Geometry: final body of the model. Coordinates: model frame, mm. A direction names the side the tool comes from. Give positions to 0.01 mm unless a question says otherwise; leave off trailing zeros. Order: outer loops, then holes, each group sorted by start corner. A loop starts at its lowest first (then second) coordinate and runs counter-clockwise, first axis right, second up. Notation, with made-up numbers: (35.5, 73) - (70.5, 73) arc R8 ccw to (70.5, 80) - close; hole circle Ø5 at (60.5, -27.75). An arc over 180 degrees is marked (long way). One line per question, with ' | ' between items. Start each with the question number.
Autodesk Fusion 360 part; units mm, degrees
sketch "Sketch1" plane through (0, 0, 0) normal (0, 1, 0) x (1, 0, 0)
  line L0 (30, 40) -> (-120, 40)
  line L1 (-120, 40) -> (-120, 20)
  line L2 (-120, 20) -> (-30, 20)
  line L3 (-30, 20) -> (-30, 0)
  arc A0 (-30, 0) -> (30, 0) centre (0, 0) ccw
  line L4 (30, 0) -> (30, 40)
  dimension "d3" = 30
  dimension "d4" = 150
  dimension "d5" = 20
  dimension "d6" = 40
extrude "Extrude1" add sketch "Sketch1" along normal blind 100
fillet "Fillet1" radius 4 1 edges at (-30, 50, -20)
sketch "Sketch2" plane through (0, 0, 0) normal (0, -1, 0) x (1, 0, 0)
  line L0 (30, -40) -> (30, 0)
  arc A0 (30, 0) -> (-30, 0) centre (0, 0) ccw
  line L1 (-30, 0) -> (-30, -16)
  arc A1 (-34, -20) -> (-30, -16) centre (-34, -16) ccw
  line L2 (-34, -20) -> (-120, -20)
  line L3 (-120, -20) -> (-120, -40)
  line L4 (-120, -40) -> (30, -40)
  circle A2 centre (0, 0) radius 15
  dimension "d10" = 30
extrude "Extrude2" cut sketch "Sketch2" against normal blind 100 contours A2
(1) Cut plane A-A, the plane x = 0. Return the cut outline in (y, z), plus the area to 3 significant figures.
(2) Pull-direction query (Z, two-part tool) for faces 1 (the cylindrical face through (-14.985, 49.3, 0.66)), 2 (the cylindrical face through (-31.141, 50.7, -18.797)), 3 (the flat face through (-29, 0, -13)); classes: +Z half, -Z half, draft (parallel to the pull), parting line (faces both ways), or undercut.
(3) Cut plane D-D, the plane x = -58. Return the cut outline in (y, z).
(4) Material intervals for line 1 along Z through (x, y) = (0, 56.5); line 2 along Z through (x, y) = (-106, 59); line 3 along X through (y, z) = (84.5, 3), sorted ascending. Write a range as from..to.
(5) Access query for faces 4 (the flat face through (-120, 49, -30)), 5 (the flat face through (-78, 49, -20)). Directions: +Z, -Z, +X, -X, +Y, -Y. A direction counts if a zero-diameter tool reaches every point of the face in a straight line with its end or side. Return the directions, or none.
(6) Contact query for flat-ended pins moving along their axis: P1, Ø1.5, axis at y = 56.5, z = 2, coming from the +X side; P2, Ø1.5, axis at x = -103, y = 33.5, coming from the +Z side; P3, Ø1.5, axis at y = 50.5, z = 8.5, coming from the +X side. Output: stop coordinate, or through.
(7) Cut plane B-B, the plane y = 83. Return the cut outline in (x, z).
(8) Cut plane C-C, the plane z = -5. Return the cut outline in (x, y).
Results are:
1) outline: (0, -40) - (100, -40) - (100, -15) - (0, -15) - close; (0, 15) - (100, 15) - (100, 30) - (0, 30) - close | area: 4,000 mm2
2) face 1: undercut | face 2: +Z half | face 3: draft
3) outline: (0, -40) - (100, -40) - (100, -20) - (0, -20) - close
4) line 1: -40..-15, 15..30 | line 2: -40..-20 | line 3: -29.85..-14.7, 14.7..29.85
5) face 4: +Z, -Z, -X, +Y, -Y | face 5: +Z, -X, +Y, -Y
6) P1: x = 29.97 | P2: z = -20 | P3: x = 28.98
7) outline: (-120, -40) - (30, -40) - (30, 0) arc R30 ccw to (-30, 0) - (-30, -16) arc R4 cw to (-34, -20) - (-120, -20) - close; hole circle Ø30 at (0, 0)
8) outline: (-30, 0) - (-14.14, 0) - (-14.14, 100) - (-30, 100) - close; (14.14, 0) - (30, 0) - (30, 100) - (14.14, 100) - close
